Work out the finished part from the listing and answer in its coordinate system (mm). Face numbers are marked on the shaded views. A direction names the side the tool comes from. Give positions to 0.01 mm unless a question says otherwise; leave off trailing zeros. Loops run counter-clockwise (first coordinate to the right, second up) from the corner with the lowest first, then second, coordinate; pieces in that order, holes last. Notation, with made-up numbers: M -19.75,26 L 30.25,26 A30 ccw 30.25,48 Z; hole C 78,26 d7. An arc over 180 degrees is marked long. Use a Markdown table: item, result.
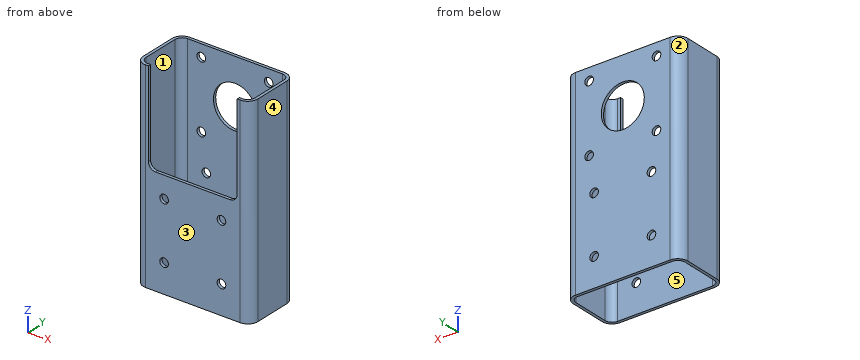
```python
from build123d import *

# Parameters (mm, degrees)
AUFSATZ_LINEAR_AUSTRAGEN1_DEPTH = 140
SKIZZE2_R                       = 15
SCHNITT_LINEAR_AUSTRAGEN1_DEPTH = 10
SCHNITT_LINEAR_AUSTRAGEN2_DEPTH = 10
SKIZZE4_R                       = 3
SCHNITT_LINEAR_AUSTRAGEN3_DEPTH = 10
SKIZZE5_R                       = 3
SCHNITT_LINEAR_AUSTRAGEN4_DEPTH = 60


with BuildPart() as part:
    # Skizze1 → Aufsatz-Linear austragen1 (new body)
    with BuildSketch(Plane.XY):
        with BuildLine():
            Line((78, 5), (78, 31))
            ThreePointArc((78, 31), (75.949747468, 35.949747468), (71, 38))
            Line((71, 38), (5, 38))
            ThreePointArc((5, 38), (0.050252532, 35.949747468), (-2, 31))
            Line((-2, 31), (-2, 5))
            ThreePointArc((-2, 5), (0.050252532, 0.050252532), (5, -2))
            Line((5, -2), (71, -2))
            ThreePointArc((71, -2), (75.949747468, 0.050252532), (78, 5))
        make_face()
        with BuildLine():
            Line((0, 31), (0, 5))
            ThreePointArc((0, 5), (1.464466094, 1.464466094), (5, 0))
            Line((5, 0), (71, 0))
            ThreePointArc((71, 0), (74.535533906, 1.464466094), (76, 5))
            Line((76, 5), (76, 31))
            ThreePointArc((76, 31), (74.535533906, 34.535533906), (71, 36))
            Line((71, 36), (5, 36))
            ThreePointArc((5, 36), (1.464466094, 34.535533906), (0, 31))
        make_face(mode=Mode.SUBTRACT)
    extrude(amount=AUFSATZ_LINEAR_AUSTRAGEN1_DEPTH)

    # Skizze2 → Schnitt-Linear austragen1 (cut)
    with BuildSketch(Plane(origin=(0, 38, 0), x_dir=(-1, 0, 0), z_dir=(0, 1, 0))):
        with Locations(Location((-38, 108, 0), (0, 0, 90))):
            Circle(SKIZZE2_R)
    extrude(amount=-SCHNITT_LINEAR_AUSTRAGEN1_DEPTH, mode=Mode.SUBTRACT)

    # Skizze3 → Schnitt-Linear austragen2 (cut)
    with BuildSketch(Plane.XZ.offset(2)):
        with BuildLine():
            Line((7, 140), (69, 140))
            Line((69, 140), (69, 80))
            ThreePointArc((69, 80), (67.535533906, 76.464466094), (64, 75))
            Line((64, 75), (12, 75))
            ThreePointArc((12, 75), (8.464466094, 76.464466094), (7, 80))
            Line((7, 80), (7, 140))
        make_face()
    extrude(amount=-SCHNITT_LINEAR_AUSTRAGEN2_DEPTH, mode=Mode.SUBTRACT)

    # Skizze4 → Schnitt-Linear austragen3 (cut)
    with BuildSketch(Plane(origin=(0, 38, 0), x_dir=(1, 0, 0), z_dir=(0, 1, 0))):
        with Locations(Location((61.5, -84.5, 0), (0, 0, 270))):
            Circle(SKIZZE4_R)
        with Locations((14.5, -84.5)):
            Circle(SKIZZE4_R)
        with Locations(Location((14.5, -131.5, 0), (0, 0, 270))):
            Circle(SKIZZE4_R)
        with Locations((61.5, -131.5)):
            Circle(SKIZZE4_R)
    extrude(amount=-SCHNITT_LINEAR_AUSTRAGEN3_DEPTH, mode=Mode.SUBTRACT)

    # Skizze5 → Schnitt-Linear austragen4 (cut)
    with BuildSketch(Plane(origin=(0, 38, 0), x_dir=(1, 0, 0), z_dir=(0, 1, 0))):
        with Locations(Location((58, -20, 0), (0, 0, 180))):
            Circle(SKIZZE5_R)
        with Locations(Location((18, -20, 0), (0, 0, 180))):
            Circle(SKIZZE5_R)
        with Locations(Location((58, -60, 0), (0, 0, 180))):
            Circle(SKIZZE5_R)
        with Locations(Location((18, -60, 0), (0, 0, 180))):
            Circle(SKIZZE5_R)
    extrude(amount=-SCHNITT_LINEAR_AUSTRAGEN4_DEPTH, mode=Mode.SUBTRACT)


solid = part.part
```
(1) The mould has two halves that part along X. Classify the marked faces 3, 4 and 5: released by +X, released by -X, zero draft, split by the parting line, or undercut.
Entries:
| item | result |
|---|---|
| face 3 | zero draft |
| face 4 | released by +X |
| face 5 | undercut |
(2) A cutting plane is placed at D-D (x = 9). Write down the section's boundary in (y, z), and give its area (3 significant figures).
Entries:
| item | result |
|---|---|
| outline | M -2,0 L 0,0 L 0,76 L -2,76 Z; M 36,0 L 38,0 L 38,140 L 36,140 Z |
| area | 432 mm² |
(3) A cutting plane is placed at C-C (x = 38). Write down the section's boundary in (y, z), and give its area (3 significant figures).
Entries:
| item | result |
|---|---|
| outline | M -2,0 L 0,0 L 0,75 L -2,75 Z; M 36,0 L 38,0 L 38,93 L 36,93 Z; M 36,123 L 38,123 L 38,140 L 36,140 Z |
| area | 370 mm² |
(4) A cutting plane is placed at A-A (y = 20). Write down the section's boundary in (x, z).
Entries:
| item | result |
|---|---|
| outline | M -2,0 L 0,0 L 0,140 L -2,140 Z; M 76,0 L 78,0 L 78,140 L 76,140 Z |
(5) Consider probe 1 along Z at (x, y) = (58, 36.9); probe 2 along Y at (x, z) = (40.5, 58); probe 3 along Z at (x, y) = (14, 37). Determine where each line is inside the solid, lowest interval first. Write a range as [from, to].
Entries:
| item | result |
|---|---|
| probe 1 | z = [0, 17], [23, 57], [63, 140] |
| probe 2 | y = [-2, 0], [36, 38] |
| probe 3 | z = [0, 81.54], [87.46, 128.54], [134.46, 140] |
(6) A cutting plane is placed at B-B (z = 131.5). Write down the section's boundary in (x, y), and give its area (3 significant figures).
Entries:
| item | result |
|---|---|
| outline | M -2,5 A7 ccw 5,-2 L 7,-2 L 7,0 L 5,0 A5 cw 0,5 L 0,31 A5 cw 5,36 L 11.5,36 L 11.5,38 L 5,38 A7 ccw -2,31 Z; M 17.5,36 L 58.5,36 L 58.5,38 L 17.5,38 Z; M 64.5,36 L 71,36 A5 cw 76,31 L 76,5 A5 cw 71,0 L 69,0 L 69,-2 L 71,-2 A7 ccw 78,5 L 78,31 A7 ccw 71,38 L 64.5,38 Z |
| area | 295 mm² |
(7) Which of the six approach directions +Z, -Z, +X, -X, +Y, -Y give full straight-line access (tool end or side, diameter ignored) to the marked faces 1 and 2?
Entries:
| item | result |
|---|---|
| face 1 | +Z, -Z |
| face 2 | +Z, -Z, -X, +Y |
(8) Given P1, Ø6, axis at y = 33.5, z = 79, coming from the +X side; P2, Ø2, axis at x = 27.5, y = -1.5, coming from the +Z side; P3, Ø1.6, axis at y = -1, z = 118, coming from the +X side; P4, Ø8, axis at x = 14.5, z = 84.5, coming from the -Y side, each flat-ended and moving along its own axis, determine where each tip first touches the part or whether it passes through.
Entries:
| item | result |
|---|---|
| P1 | stops at x = 78 |
| P2 | stops at z = 75 |
| P3 | stops at x = 75.69 |
| P4 | stops at y = 36 |
